Part print with two shaded views. Sizes in mm from the minimum x, y, z corner. Coordinates: 2 decimals unless noted, no trailing zeros. Order: outer loops, then holes, each group sorted by start corner. A loop starts at its lowest first (then second) coordinate and runs counter-clockwise, first axis right, second up. Notation, with made-up numbers: (21, 7.5) - (30, 7.5) arc R25 cw to (30, 39.5) - close; hole circle Ø4 at (6.25, -27.5). An arc over 180 degrees is marked (long way). Write each question's results on one line, items separated by ' | '. Start each with the question number.
Q1. Band-saw the part on B-B, the plane x = 57. Write the cut outline in (y, z), then the cut area to 3 significant figures.
Q2. Band-saw the part on C-C, the plane x = 34.5. Write the cut outline in (y, z), then the cut area to 3 significant figures.
Q3. Pin check, flat tips, straight feed: P1, Ø9, axis at x = 57, y = 105, coming from the +Z side; P2, Ø1.3, axis at y = 133, z = 3, coming from the -X side; P3, Ø3, axis at y = 138.5, z = 2, coming from the -X side. Stop position of each tip, or through.
Q4. Band-saw the part on A-A, the plane y = 10.5. Write the cut outline in (x, z), then the cut area to 3 significant figures.
Q5. Band-saw the part on D-D, the plane y = 105. Write the cut outline in (x, z).
Q6. Wall check: probe 1 along Y at (x, z) = (15, 1.5); probe 2 along Y at (x, z) = (5.5, 0.8); probe 3 along X at (y, z) = (42.5, 3.75). Give the ranges that are in metal, low to high.
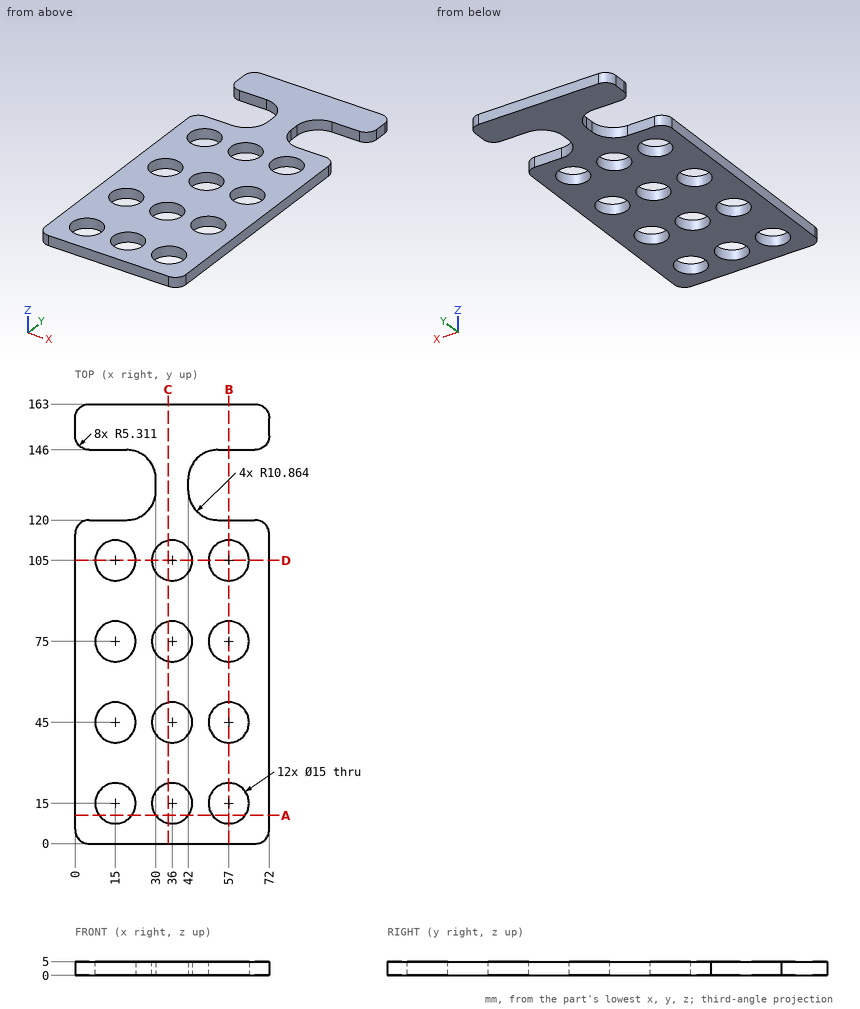
Results below:
1) outline: (0, 0) - (7.5, 0) - (7.5, 5) - (0, 5) - close; (22.5, 0) - (37.5, 0) - (37.5, 5) - (22.5, 5) - close; (52.5, 0) - (67.5, 0) - (67.5, 5) - (52.5, 5) - close; (82.5, 0) - (97.5, 0) - (97.5, 5) - (82.5, 5) - close; (112.5, 0) - (120, 0) - (120, 5) - (112.5, 5) - close; (146, 0) - (163, 0) - (163, 5) - (146, 5) - close | area: 385 mm²
2) outline: (0, 0) - (7.65, 0) - (7.65, 5) - (0, 5) - close; (22.35, 0) - (37.65, 0) - (37.65, 5) - (22.35, 5) - close; (52.35, 0) - (67.65, 0) - (67.65, 5) - (52.35, 5) - close; (82.35, 0) - (97.65, 0) - (97.65, 5) - (82.35, 5) - close; (112.35, 0) - (163, 0) - (163, 5) - (112.35, 5) - close | area: 521 mm²
3) P1: passes through | P2: stops at x = 30 | P3: stops at x = 28.85
4) outline: (0, 0) - (9, 0) - (9, 5) - (0, 5) - close; (21, 0) - (30, 0) - (30, 5) - (21, 5) - close; (42, 0) - (51, 0) - (51, 5) - (42, 5) - close; (63, 0) - (72, 0) - (72, 5) - (63, 5) - close | area: 180 mm²
5) outline: (0, 0) - (7.5, 0) - (7.5, 5) - (0, 5) - close; (22.5, 0) - (28.5, 0) - (28.5, 5) - (22.5, 5) - close; (43.5, 0) - (49.5, 0) - (49.5, 5) - (43.5, 5) - close; (64.5, 0) - (72, 0) - (72, 5) - (64.5, 5) - close
6) probe 1: y = 0 to 7.5, 22.5 to 37.5, 52.5 to 67.5, 82.5 to 97.5, 112.5 to 120, 146 to 163 | probe 2: y = 0 to 120, 146 to 163 | probe 3: x = 0 to 7.93, 22.07 to 28.93, 43.07 to 49.93, 64.07 to 72
